Autodesk Inventor part; units mm, degrees
ref_plane "YZ Plane" through (0, 0, 0) normal (1, 0, 0) x (0, 1, 0)
ref_plane "XZ Plane" through (0, 0, 0) normal (0, 1, 0) x (-1, 0, 0)
ref_plane "XY Plane" through (0, 0, 0) normal (0, 0, 1) x (1, 0, 0)
sketch "スケッチ1" plane through (0, 0, 0) normal (0, 0, 1) x (1, 0, 0)
  circle A0 centre (0, 0) radius 46.9412
  dimension "d3" = 93.8824
extrude "押し出し1" add sketch "スケッチ1" along normal blind 10.5
sketch "スケッチ2" plane through (0, 0, 10.5) normal (0, 0, 1) x (1, 0, 0)
  circle A0 centre (0, 0) radius 46.9412
  arc A1 (-5.0225, 35.5945) -> (35.5945, -5.0225) centre (0, 0) ccw
  arc A2 (35.7361, 3.8892) -> (3.8892, 35.7361) centre (0, 0) ccw
  circle A3 centre (29.2617, 29.2617) radius 2.1
  circle A4 centre (-39.9723, 10.7105) radius 2.1
  circle A5 centre (10.7105, -39.9723) radius 2.1
  circle A6 centre (0, 0) radius 35.9471
  dimension "d4" = 4.2
extrude "押し出し2" cut sketch "スケッチ2" against normal blind 5 contours A6 A2 A1
sketch "スケッチ3" plane through (0, 0, 10.5) normal (0, 0, 1) x (1, 0, 0)
  circle A0 centre (0, 0) radius 46.9412
  arc A1 (-5.0225, 35.5945) -> (35.5945, -5.0225) centre (0, 0) ccw
  arc A2 (35.7361, 3.8892) -> (3.8892, 35.7361) centre (0, 0) ccw
  circle A3 centre (29.2617, 29.2617) radius 2.1
  circle A4 centre (-39.9723, 10.7105) radius 2.1
  circle A5 centre (10.7105, -39.9723) radius 2.1
  circle A6 centre (0, 0) radius 35.9471
  dimension "d7" = 4.2
extrude "押し出し3" cut sketch "スケッチ3" against normal blind 10.5 contours A3 | A4 | A5
sketch "スケッチ4" plane through (0, 0, 5.5) normal (0, 0, 1) x (1, 0, 0)
  circle A0 centre (0, 0) radius 10.5
  circle A1 centre (0, 0) radius 10.5
extrude "押し出し4" cut sketch "スケッチ4" against normal blind 10.5
properties part number "fix_plate"
Could you check a few things on this model? Use its own coordinates, in mm. A direction names the side the tool comes from. Round coordinates to 2 decimals unless told otherwise and drop trailing zeros. Write each loop counter-clockwise with the first axis right and the second up, starting at its lowest first coordinate (ties: lowest second). Pieces come first, ordered by that corner, then holes. Notation, with made-up numbers: (-23, 19) - (-18, 19) arc R12 ccw to (-18, 35) - close; hole circle Ø2 at (31, 28). An arc over 180 degrees is marked (long way). Use a Markdown table: item, result.
Q1. I want a section at A-A (y = 0). List the corners of the cut face in (x, z) for me, plus the area to 3 significant figures.
Output values:
| item | result |
|---|---|
| outline | (-46.94, 0) - (-10.5, 0) - (-10.5, 5.5) - (-35.95, 5.5) - (-35.95, 10.5) - (-46.94, 10.5) - close; (10.5, 0) - (46.94, 0) - (46.94, 10.5) - (35.95, 10.5) - (35.95, 5.5) - (10.5, 5.5) - close |
| area | 511 mm2 |
Q2. Please list where these lines run through material, in increasing order: L1, parallel to X at y = 9, z = 5; L2, parallel to Y at x = 0, z = 9.3; L3, parallel to X at y = 1, z = 10.
Output values:
| item | result |
|---|---|
| L1 | -46.07 to -41.19, -38.75 to -5.41, 5.41 to 46.07 |
| L2 | -46.94 to -35.95, 35.95 to 46.94 |
| L3 | -46.93 to -35.93, 35.93 to 46.93 |
Q3. Thinking about a two-plate mould opening in Y: for faces 1 (the cylindrical face through (-6.11, -46.54, 5.18)), 2 (the cylindrical face through (25.658, 25.176, 8.035)), 3 (the flat face through (10, -35, 10.5)), 4 (the cylindrical face through (-40.2, 12.8, 5.3)), which applies, released by +Y, released by -Y, zero draft, split by the parting line, or undercut?
Output values:
| item | result |
|---|---|
| face 1 | split by the parting line |
| face 2 | undercut |
| face 3 | zero draft |
| face 4 | undercut |
Q4. For faces 5 (the flat face through (-1, 11, 0)), 6 (the flat face through (-8.5, -7.5, 5.5)), which set-ups out of +Z, -Z, +X, -X, +Y, -Y let a thin tool reach every point of the face, with its end or its side?
Output values:
| item | result |
|---|---|
| face 5 | -Z, +X, -X, +Y, -Y |
| face 6 | +Z |
Q5. For pin 1 (2 mm diameter, centred on x = 31.5, z = 7, fed in from +Y); pin 2 (2 mm diameter, centred on y = 3.5, z = 6, fed in from +X); pin 3 (1.5 mm diameter, centred on x = 24.5, y = -5, fed in from +Z), each with a flat end and sliding along its axis, tell me the tip position at first contact or that it passes through.
Output values:
| item | result |
|---|---|
| pin 1 | y = 35.68 |
| pin 2 | x = 46.87 |
| pin 3 | z = 5.5 |
Q6. I want a section at D-D (y = -25.5). List the corners of the cut face in (x, z) for me, plus the area to 3 significant figures.
Output values:
| item | result |
|---|---|
| outline | (-39.41, 0) - (39.41, 0) - (39.41, 10.5) - (25.34, 10.5) - (25.34, 5.5) - (-25.34, 5.5) - (-25.34, 10.5) - (-39.41, 10.5) - close |
| area | 574 mm2 |
Q7. I want a section at C-C (z = 2.25). List the corners of the cut face in (x, y) for me, plus the area to 3 significant figures.
Output values:
| item | result |
|---|---|
| outline | circle Ø93.88 at (0, 0); hole circle Ø4.2 at (-39.97, 10.71); hole circle Ø21 at (0, 0); hole circle Ø4.2 at (10.71, -39.97); hole circle Ø4.2 at (29.26, 29.26) |
| area | 6,530 mm2 |
